Verification items for the finished model (mm, model axes). A direction names the side the tool comes from. Coordinates: 2 decimals unless noted, no trailing zeros. Write each loop counter-clockwise with the first axis right and the second up, starting at its lowest first coordinate (ties: lowest second). Pieces come first, ordered by that corner, then holes. Notation, with made-up numbers: M 72,56.5 L 94,56.5 A28 cw 94,84.5 Z; hole C 26,-32.75 d2. An arc over 180 degrees is marked long. One line per item, written item: value.
```python
from build123d import *

# Parameters (mm, degrees)
SKETCH1_R           = 1.6
BOSS_EXTRUDE1_DEPTH = 3
FILLET1_R           = 2
FILLET2_R           = 5


with BuildPart() as part:
    # Sketch1 → Boss-Extrude1 (new body)
    with BuildSketch(Plane(origin=(0, 0, 0), x_dir=(1, 0, 0), z_dir=(0, 1, 0))):
        with BuildLine():
            Line((-126.554445662, 87.5), (-104.054445662, 87.5))
            Line((-104.054445662, 87.5), (-104.054445662, 77.5))
            Line((-104.054445662, 77.5), (-114.054445662, 67.5))
            Line((-114.054445662, 67.5), (-114.054445662, 57.5))
            Line((-114.054445662, 57.5), (-94.037011093, 37.482565431))
            Line((-94.037011093, 37.482565431), (-66.537011093, 37.482565431))
            Line((-66.537011093, 37.482565431), (-56.537011093, 37.482565431))
            Line((-56.537011093, 37.482565431), (-29.037011093, 37.482565431))
            Line((-29.037011093, 37.482565431), (-9.054445662, 57.465130862))
            Line((-9.054445662, 57.465130862), (-9.054445662, 67.5))
            Line((-9.054445662, 67.5), (-19.054445662, 77.5))
            Line((-19.054445662, 77.5), (-19.054445662, 87.5))
            Line((-19.054445662, 87.5), (37.5, 87.5))
            Line((37.5, 87.5), (37.5, 77.5))
            Line((37.5, 77.5), (27.5, 67.5))
            Line((27.5, 67.5), (27.5, 57.5))
            Line((27.5, 57.5), (47.5, 37.5))
            Line((47.5, 37.5), (72.157583055, 37.5))
            Line((72.157583055, 37.5), (87.842416945, 37.5))
            Line((87.842416945, 37.5), (112.5, 37.5))
            Line((112.5, 37.5), (132.5, 57.5))
            Line((132.5, 57.5), (132.5, 67.5))
            Line((132.5, 67.5), (122.5, 77.5))
            Line((122.5, 77.5), (122.5, 87.5))
            Line((122.5, 87.5), (136.956007081, 87.5))
            Line((136.956007081, 87.5), (145.020423476, 87.5))
            ThreePointArc((145.020423476, 87.5), (168.465977814, 0), (145.020423476, -87.5))
            Line((145.020423476, -87.5), (136.956007081, -87.5))
            Line((136.956007081, -87.5), (122.5, -87.5))
            Line((122.5, -87.5), (122.5, -77.5))
            Line((122.5, -77.5), (132.5, -67.5))
            Line((132.5, -67.5), (132.5, -57.5))
            Line((132.5, -57.5), (112.5, -37.5))
            Line((112.5, -37.5), (87.842416945, -37.5))
            Line((87.842416945, -37.5), (72.157583055, -37.5))
            Line((72.157583055, -37.5), (47.5, -37.5))
            Line((47.5, -37.5), (27.5, -57.5))
            Line((27.5, -57.5), (27.5, -67.5))
            Line((27.5, -67.5), (37.5, -77.5))
            Line((37.5, -77.5), (37.5, -87.5))
            Line((37.5, -87.5), (-19.054445662, -87.5))
            Line((-19.054445662, -87.5), (-19.054445662, -77.5))
            Line((-19.054445662, -77.5), (-9.054445662, -67.5))
            Line((-9.054445662, -67.5), (-9.054445662, -57.465130862))
            Line((-9.054445662, -57.465130862), (-29.037011093, -37.482565431))
            Line((-29.037011093, -37.482565431), (-56.537011093, -37.482565431))
            Line((-56.537011093, -37.482565431), (-66.537011093, -37.482565431))
            Line((-66.537011093, -37.482565431), (-94.037011093, -37.482565431))
            Line((-94.037011093, -37.482565431), (-114.054445662, -57.5))
            Line((-114.054445662, -57.5), (-114.054445662, -67.5))
            Line((-114.054445662, -67.5), (-104.054445662, -77.5))
            Line((-104.054445662, -77.5), (-104.054445662, -87.5))
            Line((-104.054445662, -87.5), (-126.554445662, -87.5))
            ThreePointArc((-126.554445662, -87.5), (-150, 0), (-126.554445662, 87.5))
        make_face()
        with Locations((-125, -30)):
            Circle(SKETCH1_R, mode=Mode.SUBTRACT)
        with Locations((9.232988907, -36)):
            Circle(SKETCH1_R, mode=Mode.SUBTRACT)
        with Locations((143.46, -30)):
            Circle(SKETCH1_R, mode=Mode.SUBTRACT)
        with Locations((143.46, 30)):
            Circle(SKETCH1_R, mode=Mode.SUBTRACT)
        with Locations((9.232988907, 36)):
            Circle(SKETCH1_R, mode=Mode.SUBTRACT)
        with Locations((-125, 30)):
            Circle(SKETCH1_R, mode=Mode.SUBTRACT)
    extrude(amount=BOSS_EXTRUDE1_DEPTH)

    # Fillet1
    fillet1_edges = [part.edges().sort_by_distance(p)[0] for p in [
        (-104.054445662, 1.5, 87.5),
        (-104.054445662, 1.5, -87.5),
        (-104.054445662, 1.5, -77.5),
        (-114.054445662, 1.5, -67.5),
        (-114.054445662, 1.5, -57.5),
        (-94.037011093, 1.5, -37.482565431),
        (-29.037011093, 1.5, -37.482565431),
        (-9.054445662, 1.5, -57.465130862),
        (-9.054445662, 1.5, -67.5),
        (-19.054445662, 1.5, -77.5),
        (-19.054445662, 1.5, -87.5),
        (37.5, 1.5, -87.5),
        (37.5, 1.5, -77.5),
        (27.5, 1.5, -67.5),
        (27.5, 1.5, -57.5),
        (47.5, 1.5, -37.5),
        (112.5, 1.5, -37.5),
        (132.5, 1.5, -57.5),
        (132.5, 1.5, -67.5),
        (122.5, 1.5, -77.5),
        (122.5, 1.5, -87.5),
        (122.5, 1.5, 87.5),
        (122.5, 1.5, 77.5),
        (132.5, 1.5, 67.5),
        (132.5, 1.5, 57.5),
        (112.5, 1.5, 37.5),
        (47.5, 1.5, 37.5),
        (27.5, 1.5, 57.5),
        (27.5, 1.5, 67.5),
        (37.5, 1.5, 77.5),
        (37.5, 1.5, 87.5),
        (-19.054445662, 1.5, 87.5),
        (-19.054445662, 1.5, 77.5),
        (-9.054445662, 1.5, 67.5),
        (-9.054445662, 1.5, 57.465130862),
        (-29.037011093, 1.5, 37.482565431),
        (-94.037011093, 1.5, 37.482565431),
        (-114.054445662, 1.5, 57.5),
        (-114.054445662, 1.5, 67.5),
        (-104.054445662, 1.5, 77.5),
    ]]
    fillet(fillet1_edges, radius=FILLET1_R)

    # Fillet2
    fillet2_edges = [part.edges().sort_by_distance(p)[0] for p in [
        (-126.554445662, 1.5, 87.5),
        (-126.554445662, 1.5, -87.5),
        (145.020423476, 1.5, -87.5),
        (145.020423476, 1.5, 87.5),
    ]]
    fillet(fillet2_edges, radius=FILLET2_R)


solid = part.part
```
Item 1: Cross-section at B-B, the plane y = 2.55. Give the number of separate pieces and of enclosed holes in the cut face, and give its area (3 significant figures).
The answers:
separate pieces: 1
enclosed holes: 6
area: 34,800 mm²
Item 2: Access from +Z, -Z, +X, -X, +Y, -Y to the whole of each face (thin tool, end or side, straight path). Record for faces 4 (the face through (37, 1, -48)), 5 (the face through (-149.996, 1.479, 1.241)).
The answers:
face 4: +Y, -Y
face 5: -X, +Y, -Y
Item 3: Go/stop test with flat-tipped pins: P1, Ø0.9, axis at y = 1, z = 80.5, coming from the +X side; P2, Ø1.5, axis at y = 2, z = 21.5, coming from the -X side; P3, Ø0.9, axis at y = 1, z = 64, coming from the +X side. Record where each tip stops, or that it passes through.
The answers:
P1: stops at x = 149.08
P2: stops at x = -148.77
P3: stops at x = 156.52
Item 4: Cross-section at C-C, the plane x = 94. Enter the section's corners in (y, z).
The answers:
outline: M 0,-37.5 L 3,-37.5 L 3,37.5 L 0,37.5 Z
Item 5: Cross-section at A-A, the plane x = 128. Enter the section's corners in (y, z).
The answers:
outline: M 0,-87.5 L 3,-87.5 L 3,-72 L 0,-72 Z; M 0,-53 L 3,-53 L 3,53 L 0,53 Z; M 0,72 L 3,72 L 3,87.5 L 0,87.5 Z
Item 6: Scan lines: line 1 (X direction, y = 0.9, z = 57); line 2 (Z direction, x = 31, y = 1.95); line 3 (Z direction, x = -9.5, y = 2.7). Record each from-to range of solid material in increasing order.
The answers:
line 1: x = -140.46 to -113.55, -9.53 to 28, 132 to 158.92
line 2: z = -87.5 to -71, -54 to 54, 71 to 87.5
line 3: z = -87.5 to -67.93, -57.04 to 57.04, 67.93 to 87.5
Item 7: Draft check along X on faces 1 (the face through (11, 3, -1)), 2 (the face through (168.46, 1.48, -1.24)), 3 (the face through (32, 1, 72)). Enter one of: released by +X, released by -X, zero draft, split by the parting line, or undercut.
The answers:
face 1: zero draft
face 2: released by +X
face 3: undercut
